CAD build for the part. Positions are in the model's coordinates, mm. Coordinates: 2 decimals unless noted, no trailing zeros. Loops run counter-clockwise (first coordinate to the right, second up) from the corner with the lowest first, then second, coordinate; pieces in that order, holes last.
1) Saw through at C-C, the plane y = -10.5. Give the number of separate pieces and of enclosed holes in the cut face, and give its area (3 significant figures).
2) Saw through at B-B, the plane x = -292.1. Write the cut outline in (y, z).
3) Pin check, flat tips, straight feed: pin 1 Ø4 at (y, z) = (-9.5, 28) entering from +X; pin 2 Ø3 at (y, z) = (-5.5, 63.5) entering from +X; pin 3 Ø7 at (y, z) = (-10.5, -4) entering from +X (3 decimals). Stop position of each tip, or through.
4) Saw through at A-A, the plane x = 259.5. Write the cut outline in (y, z).
5) Wall check: line 1 along X through (y, z) = (-3.5, -82); line 2 along X through (y, z) = (-1.25, -5); line 3 along Z through (x, y) = (283, -13). Give the ranges that are in metal, low to high.
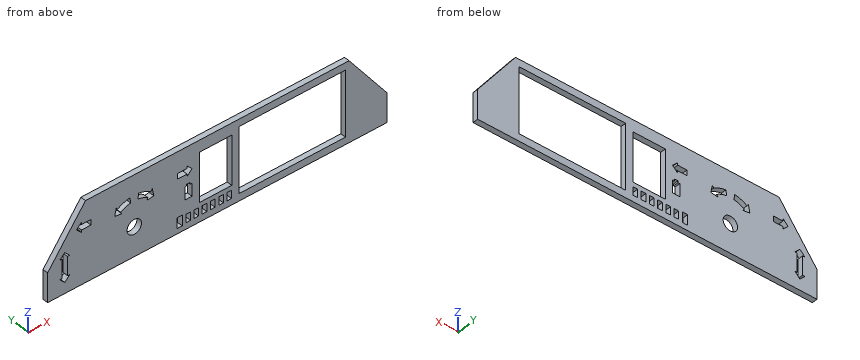
```python
from build123d import *

# Parameters (mm, degrees)
F0_W     = 16.002
F0_H     = 28.575
F0_W_2   = 16.383
F0_R     = 25.4
F0_W_3   = 114.3
F0_H_2   = 171.45
F1_DEPTH = 19.05


with BuildPart() as f1:
    # F0 (on Front) → F1 (new body)
    with BuildSketch(Plane.XZ):
        Polygon((-596.9, -50.8), (-596.9, -127), (-596.9, -152.4), (596.9, -152.4), (596.9, -127), (596.9, -50.8), (463.55, 127), (-463.55, 127), align=None)
        Polygon((-123.19, -97.549498), (-123.19, -101.6), (-123.19, -115.8875), (-123.19, -130.175), (-123.19, -134.215891), (-142.208517, -134.215891), (-142.208517, -97.549498), align=None, mode=Mode.SUBTRACT)
        with Locations((-102.489, -115.8875)):
            Rectangle(F0_W, F0_H, mode=Mode.SUBTRACT)
        with Locations((-73.787, -115.8875)):
            Rectangle(F0_W, F0_H, mode=Mode.SUBTRACT)
        with Locations((-44.8945, -115.8875)):
            Rectangle(F0_W_2, F0_H, mode=Mode.SUBTRACT)
        with Locations((-15.8115, -115.8875)):
            Rectangle(F0_W_2, F0_H, mode=Mode.SUBTRACT)
        Polygon((-518.614488, -96.339488), (-536.575, -114.3), (-554.535512, -96.339488), (-546.1, -96.339488), (-546.1, -63.5), (-546.1, -30.660512), (-554.535512, -30.660512), (-536.575, -12.7), (-518.614488, -30.660512), (-527.05, -30.660512), (-527.05, -63.5), (-527.05, -96.339488), align=None, mode=Mode.SUBTRACT)
        with Locations((-292.1, -50.8)):
            Circle(F0_R, mode=Mode.SUBTRACT)
        Polygon((-88.9, -50.8), (-114.3, -50.8), (-114.3, -6.35), (-107.95, -6.35), (-107.95, 0), (-95.25, 0), (-95.25, -6.35), (-88.9, -6.35), align=None, mode=Mode.SUBTRACT)
        with Locations((13.2715, -115.8875)):
            Rectangle(F0_W_2, F0_H, mode=Mode.SUBTRACT)
        with Locations((42.164, -115.8875)):
            Rectangle(F0_W, F0_H, mode=Mode.SUBTRACT)
        Polygon((450.85, -127), (76.2, -127), (76.2, 101.6), (450.85, 101.6), (450.85, 0), align=None, mode=Mode.SUBTRACT)
        Polygon((-477.339488, 52.885512), (-444.5, 52.885512), (-444.5, 33.835512), (-477.339488, 33.835512), (-477.339488, 25.4), (-495.3, 43.360512), (-477.339488, 61.321024), align=None, mode=Mode.SUBTRACT)
        with BuildLine():
            ThreePointArc((-350.831293, 39.775039), (-330.058088, 50.256351), (-307.521429, 56.042791))
            Line((-307.521429, 56.042791), (-304.8, 37.188181))
            ThreePointArc((-304.8, 37.188181), (-323.359602, 32.422877), (-340.466947, 23.791209))
            Line((-340.466947, 23.791209), (-335.877518, 16.713419))
            Line((-335.877518, 16.713419), (-360.769437, 19.712333))
            Line((-360.769437, 19.712333), (-355.420722, 46.852828))
            Line((-355.420722, 46.852828), (-350.831293, 39.775039))
        make_face(mode=Mode.SUBTRACT)
        with Locations((-6.35, 0)):
            Rectangle(F0_W_3, F0_H_2, mode=Mode.SUBTRACT)
        with BuildLine():
            Line((-279.264106, 37.168459), (-276.513557, 56.018843))
            ThreePointArc((-276.513557, 56.018843), (-254.063875, 50.227005), (-233.368707, 39.775039))
            Line((-233.368707, 39.775039), (-228.779278, 46.852828))
            Line((-228.779278, 46.852828), (-223.430563, 19.712333))
            Line((-223.430563, 19.712333), (-248.564992, 16.876708))
            Line((-248.564992, 16.876708), (-243.733053, 23.791209))
            ThreePointArc((-243.733053, 23.791209), (-260.776133, 32.39871), (-279.264106, 37.168459))
        make_face(mode=Mode.SUBTRACT)
        Polygon((-139.534989, 33.835512), (-139.534989, 52.885512), (-106.695501, 52.885512), (-106.695501, 61.321024), (-88.734989, 43.360512), (-106.695501, 25.4), (-106.695501, 33.835512), align=None, mode=Mode.SUBTRACT)
    extrude(amount=F1_DEPTH)


solid = f1.part
```
Data:
1. separate pieces: 1
1. enclosed holes: 16
1. area: 192,000 mm2
2. outline: (-19.05, -152.4) - (0, -152.4) - (0, -76.2) - (-19.05, -76.2) - close; (-19.05, -25.4) - (0, -25.4) - (0, 127) - (-19.05, 127) - close
3. pin 1: stops at x = 539.3
3. pin 2: stops at x = 512.3
3. pin 3: stops at x = 564.425
4. outline: (-19.05, -152.4) - (0, -152.4) - (0, -127) - (-19.05, -127) - close; (-19.05, 101.6) - (0, 101.6) - (0, 127) - (-19.05, 127) - close
5. line 1: x = -596.9 to -546.1, -527.05 to -63.5, 50.8 to 76.2, 450.85 to 596.9
5. line 2: x = -562.55 to -107.95, -95.25 to -63.5, 50.8 to 76.2, 450.85 to 562.55
5. line 3: z = -152.4 to -127, 101.6 to 127
